from build123d import *

# Parameters (mm, degrees)
BOSS_EXTRUDE1_DEPTH = 60
SKETCH3_W           = 66
SKETCH3_H           = 14
BOSS_EXTRUDE2_DEPTH = 5


with BuildPart() as part:
    # Sketch1 → Boss-Extrude1 (new body)
    with BuildSketch(Plane(origin=(0, 0, 0), x_dir=(0, 0, -1), z_dir=(1, 0, 0))):
        Polygon((0, 0), (8, 8), (88, 8), (88, 0), align=None)
    extrude(amount=BOSS_EXTRUDE1_DEPTH)

    # Sketch3 → Boss-Extrude2 (add)
    with BuildSketch(Plane(origin=(0, 0, -88), x_dir=(-1, 0, 0), z_dir=(0, 0, -1))):
        with Locations((-30, 4)):
            Rectangle(SKETCH3_W, SKETCH3_H)
    extrude(amount=BOSS_EXTRUDE2_DEPTH)


solid = part.part
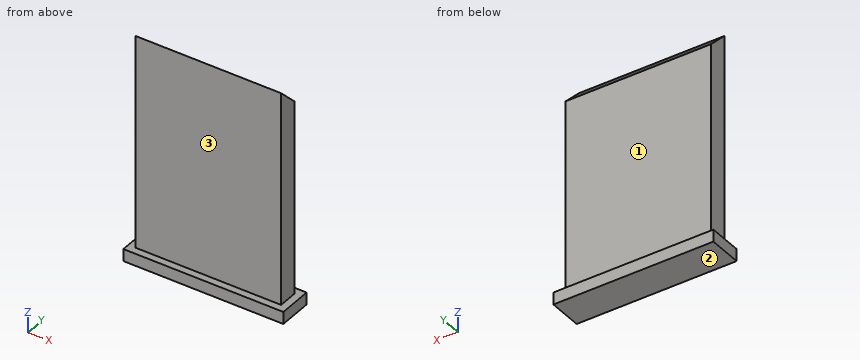
The listing builds one solid part. Answer for the finished solid, in the listing's coordinates (mm). Face numbers are marked on the shaded views. A direction names the side the tool comes from. Give positions to 0.01 mm unless a question says otherwise; leave off trailing zeros. Order: outer loops, then holes, each group sorted by start corner. A loop starts at its lowest first (then second) coordinate and runs counter-clockwise, first axis right, second up. Notation, with made-up numbers: (36, 54.5) - (56, 54.5) arc R18 cw to (56, 86.5) - close; hole circle Ø1 at (-25.5, 79). An arc over 180 degrees is marked (long way). Answer as CSV lines item,"result".
Q1. Straight lines are drawn through the part: L1, parallel to Z at x = 41.5, y = -2.25; L2, parallel to X at y = 4, z = -20; L3, parallel to Y at x = 45, z = -60.5. For each, find the intervals that lie inside material, in ascending order.
Answer key:
L1,"z = -93 to -88"
L2,"x = 0 to 60"
L3,"y = 0 to 8"
Q2. Each of these flat-tipped pins is pushed along its axis until it touches: pin 1 Ø2 at (x, y) = (10.5, 5) entering from +Z; pin 2 Ø2.5 at (y, z) = (5.5, -57) entering from +X; pin 3 Ø4 at (x, z) = (37, -44.5) entering from +Y. Where does it stop, or does it pass through?
Answer key:
pin 1,"stops at z = -4"
pin 2,"stops at x = 60"
pin 3,"stops at y = 8"
Q3. A cutting plane is placed at C-C, the plane z = -44. Determine the outline of the cut face in (x, y).
Answer key:
outline,"(0, 0) - (60, 0) - (60, 8) - (0, 8) - close"
Q4. A cutting plane is placed at A-A, the plane y = 5.75. Determine the outline of the cut face in (x, z).
Answer key:
outline,"(-3, -93) - (63, -93) - (63, -88) - (60, -88) - (60, -5.75) - (0, -5.75) - (0, -88) - (-3, -88) - close"
Q5. Which of the six approach directions +Z, -Z, +X, -X, +Y, -Y give full straight-line access (tool end or side, diameter ignored) to the marked faces 1, 2 and 3?
Answer key:
face 1,"+Z, +X, -X, +Y"
face 2,"-Z, +X, -X, +Y, -Y"
face 3,"+Z, +X, -X, -Y"
Q6. A cutting plane is placed at B-B, the plane x = 28.5. Determine the outline of the cut face in (y, z), and give its area (3 significant figures).
Answer key:
outline,"(-3, -93) - (11, -93) - (11, -88) - (8, -88) - (8, -8) - (0, 0) - (0, -88) - (-3, -88) - close"
area,"742 mm^2"
